Part model, mm, in its own coordinate system. Face numbers are marked on the shaded views. Round coordinates to 2 decimals unless told otherwise and drop trailing zeros. Loops run counter-clockwise (first coordinate to the right, second up) from the corner with the lowest first, then second, coordinate; pieces in that order, holes last. Notation, with made-up numbers: (-18.5, 48.5) -> (38.5, 48.5) arc R9 ccw to (38.5, 58.5) -> close; hole circle Ø4 at (-5.75, -15.5). An arc over 180 degrees is marked (long way). Answer as a JSON object with one key per item and string values. Group by question number.
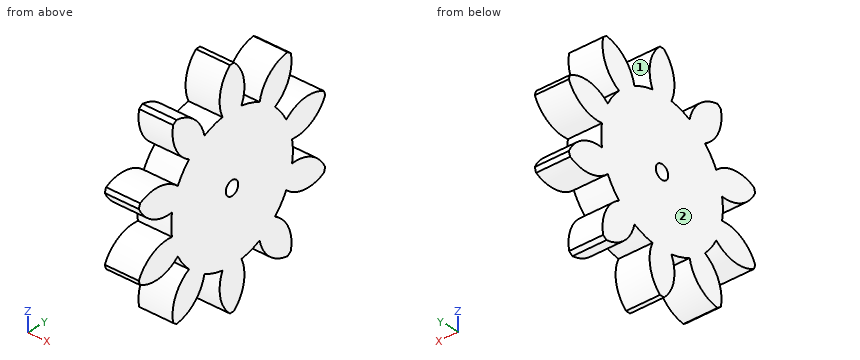
from build123d import *

# Parameters (mm, degrees)
BASPROSKE_W           = 12
BASPROSKE_H           = 39
TOOTHCUT_DEPTH        = 57.444663167
TEETHCUTS_COUNT       = 10
TEETHCUTS_ANGLE       = 324
BORSKE_R              = 1.5
BORE_DEPTH            = 50.0000508
CROQUIS1_R            = 2.5
CORTAR_EXTRUIR1_DEPTH = 56.31066802


with BuildPart() as part:
    # BasProSke → Base-Revolve (revolve)
    with BuildSketch(Plane(origin=(0, 0, 0), x_dir=(1, 0, 0), z_dir=(0, 1, 0)), mode=Mode.PRIVATE) as base_revolve_sk:
        with Locations((6, 19.5)):
            Rectangle(BASPROSKE_W, BASPROSKE_H)
    revolve(base_revolve_sk.sketch.rotate(Axis((-10, 0, 0), (1, 0, 0)), 180), axis=Axis((-10, 0, 0), (1, 0, 0)))

    # TooCutSke → ToothCut (cut, through all)
    with BuildSketch(Plane(origin=(0, 0, 0), x_dir=(0, 0, -1), z_dir=(1, 0, 0))):
        with BuildLine():
            ThreePointArc((3.815775932, 24.073465269), (0, 24.374), (-3.815775932, 24.073465269))
            ThreePointArc((-3.815775932, 24.073465269), (-5.403120307, 31.925375456), (-11.292153099, 37.355978418))
            ThreePointArc((-11.292153099, 37.355978418), (0, 39.0254), (11.292153099, 37.355978418))
            ThreePointArc((11.292153099, 37.355978418), (5.403120307, 31.925375456), (3.815775932, 24.073465269))
        make_face()
    toothcut = extrude(amount=TOOTHCUT_DEPTH, mode=Mode.SUBTRACT)

    # TeethCuts: ToothCut ×10 about axis
    teethcuts_axis = Axis((-10, 0, 0), (1, 0, 0))
    for i in range(1, TEETHCUTS_COUNT):
        add(toothcut.rotate(teethcuts_axis, i * TEETHCUTS_ANGLE / (TEETHCUTS_COUNT - 1)), mode=Mode.SUBTRACT)

    # BorSke → Bore (cut, symmetric)
    with BuildSketch(Plane(origin=(0, 0, 0), x_dir=(0, 0, -1), z_dir=(1, 0, 0))):
        with Locations(Location((0, 0, 0), (0, 0, 180))):
            Circle(BORSKE_R)
    extrude(amount=BORE_DEPTH, both=True, mode=Mode.SUBTRACT)

    # Croquis1 → Cortar-Extruir1 (cut, through all)
    with BuildSketch(Plane.YZ.offset(12)):
        with Locations(Location((0, 0, 0), (0, 0, 270))):
            Circle(CROQUIS1_R)
    extrude(amount=-CORTAR_EXTRUIR1_DEPTH, mode=Mode.SUBTRACT)


solid = part.part
Item 1: Band-saw the part on A-A, the plane z = 0. List the corners of the cut face in (x, y).
Item 2: Band-saw the part on D-D, the plane y = -7.5. List the corners of the cut face in (x, z), plus the area to 3 significant figures.
Item 3: Two-plate mould, pull along Z, no slides. Class the marked faces 1 and 2: pulls with the +Z half, pulls with the -Z half, needs draft (parallel to the pull), parting line crosses it, or undercut.
Item 4: Drill centre lines: line 1 (Y direction, x = 7.25, z = 0); line 2 (Y direction, x = 2.5, z = -28.5); line 3 (Z direction, x = 4.75, y = 21.5). Where is each one in solid material? Low to high.
Item 5: Drop flat-ended pins along their axis: pin 1 Ø4.5 at (y, z) = (0, 0) entering from -X; pin 2 Ø3 at (x, z) = (2.5, -28) entering from +Y; pin 3 Ø5 at (x, y) = (7.5, 1.5) entering from -Z; pin 4 Ø3 at (x, y) = (2.5, -25.5) entering from -Z. Give the stop position or say it passes through.
Item 6: Band-saw the part on B-B, the plane z = 29. List the corners of the cut face in (x, y), plus the area to 3 significant figures.
Item 7: Band-saw the part on C-C, the plane y = 19.5. List the corners of the cut face in (x, z), plus the area to 3 significant figures.
Entries:
{
 "1": {"outline": "(0, -24.37) -> (12, -24.37) -> (12, -2.5) -> (0, -2.5) -> close; (0, 2.5) -> (12, 2.5) -> (12, 24.37) -> (0, 24.37) -> close"},
 "2": {"outline": "(0, -23.19) -> (12, -23.19) -> (12, 23.19) -> (0, 23.19) -> close", "area": "557 mm²"},
 "3": {"face 1": "undercut", "face 2": "needs draft"},
 "4": {"line 1": "-24.37 to -2.5, 2.5 to 24.37", "line 2": "-23.83 to -14.8, -4.95 to 4.95, 14.8 to 23.83", "line 3": "-31.92 to -21.12, -11.48 to 11.48, 21.12 to 31.92"},
 "5": {"pin 1": "through", "pin 2": "y = 23.83", "pin 3": "z = -39", "pin 4": "z = -14"},
 "6": {"outline": "(0, -23.83) -> (12, -23.83) -> (12, -15.35) -> (0, -15.35) -> close; (0, -4.97) -> (12, -4.97) -> (12, 4.97) -> (0, 4.97) -> close; (0, 15.35) -> (12, 15.35) -> (12, 23.83) -> (0, 23.83) -> close", "area": "323 mm²"},
 "7": {"outline": "(0, -31.39) -> (12, -31.39) -> (12, -18.86) -> (0, -18.86) -> close; (0, -14.62) -> (12, -14.62) -> (12, 14.62) -> (0, 14.62) -> close; (0, 18.86) -> (12, 18.86) -> (12, 31.39) -> (0, 31.39) -> close", "area": "652 mm²"}
}
